```python
from build123d import *

# Parameters (mm, degrees)
F0_R     = 11.5
F1_DEPTH = 2
F2_R     = 11.5
F2_R_2   = 10.25
F3_DEPTH = 15
F4_R     = 1.25
F5_DEPTH = 15


with BuildPart() as f1:
    # F0 (on Top) → F1 (new body)
    with BuildSketch(Plane.XY):
        Circle(F0_R)
    extrude(amount=F1_DEPTH)

    # F2 (on face) → F3 (join)
    with BuildSketch(Plane.XY.offset(2)):
        Circle(F2_R)
        Circle(F2_R_2, mode=Mode.SUBTRACT)
    extrude(amount=F3_DEPTH)

    # F4 (on face) → F5 (join)
    with BuildSketch(Plane.XY.offset(2)):
        Circle(F4_R)
    extrude(amount=F5_DEPTH)


solid = f1.part
```
Design review of the part built by this model. Coordinates are the model's own, in mm. A direction names the side the tool comes from. Give positions to 0.01 mm unless a question says otherwise; leave off trailing zeros. Order: outer loops, then holes, each group sorted by start corner. A loop starts at its lowest first (then second) coordinate and runs counter-clockwise, first axis right, second up. Notation, with made-up numbers: (-36, 73) - (10, 73) arc R22 ccw to (10, 92) - close; hole circle Ø3 at (-8, -21). An arc over 180 degrees is marked (long way). Use a Markdown table: item, result. Add a question column.
(1) Clearance check with flat-ended pins moving along their axes: P1, Ø4, axis at x = 9, z = 4.5, coming from the -Y side; P2, Ø10, axis at x = -7.5, z = 6.5, coming from the +Y side (3 decimals); P3, Ø6, axis at y = -6.5, z = 4, coming from the +X side. State where each tip first meets the part, or that it passes through.
(2) Add section D-D on x = 2.5. Give the boundary of the cut face in (y, z), then the cut area to 3 significant figures.
(3) Wall thickness on probe 1 along Y at (x, z) = (0, 6); probe 2 along X at (y, z) = (0.5, 11.5); probe 3 along Z at (x, y) = (4.75, -3): over which ranges is each line inside the solid? List them lowest first. Write a range as [from, to].
(4) Mouldability with a two-part tool opening along X and no side actions: class faces 3 (the face through (2, 0, 2)), 4 (the face through (-1.5, 11.4, 8.4)), 5 (the face through (0, 0, 17)) as +X half, -X half, draft (parallel to the pull), parting line (faces both ways), or undercut.
(5) Machinability: for faces 1 (the face through (-8, -7, 17)), 2 (the face through (-0.27, -1.22, 9.4)), which of the approach directions +Z, -Z, +X, -X, +Y, -Y give a long, thin tool a straight path to every point of the face, cutting with its end or side? Answer none if there is none.
(6) Add section B-B on x = 0. Give the boundary of the cut face in (y, z).
(7) Add section A-A on z = 7.5. Give the boundary of the cut face in (x, y).
Report:
| question | item | result |
|---|---|---|
| 1 | P1 | stops at y = -9.12 |
| 1 | P2 | stops at y = 11.225 |
| 1 | P3 | stops at x = 10.95 |
| 2 | outline | (-11.22, 0) - (11.22, 0) - (11.22, 17) - (9.94, 17) - (9.94, 2) - (-9.94, 2) - (-9.94, 17) - (-11.22, 17) - close |
| 2 | area | 83.4 mm² |
| 3 | probe 1 | y = [-11.5, -10.25], [-1.25, 1.25], [10.25, 11.5] |
| 3 | probe 2 | x = [-11.49, -10.24], [-1.15, 1.15], [10.24, 11.49] |
| 3 | probe 3 | z = [0, 2] |
| 4 | face 3 | undercut |
| 4 | face 4 | parting line |
| 4 | face 5 | draft |
| 5 | face 1 | +Z, +X, -X, +Y, -Y |
| 5 | face 2 | +Z |
| 6 | outline | (-11.5, 0) - (11.5, 0) - (11.5, 17) - (10.25, 17) - (10.25, 2) - (1.25, 2) - (1.25, 17) - (-1.25, 17) - (-1.25, 2) - (-10.25, 2) - (-10.25, 17) - (-11.5, 17) - close |
| 7 | outline | circle Ø23 at (0, 0); circle Ø2.5 at (0, 0); hole circle Ø20.5 at (0, 0) |
